from build123d import *
from build123d.topology import SkipClean

# Parameters (mm, degrees)
SKETCH1_R           = 15.24
SKETCH1_R_2         = 14.01445
BOSS_EXTRUDE1_DEPTH = 19.304
SKETCH2_R           = 14.01445
CUT_EXTRUDE1_DEPTH  = 29.934204707
CUT_EXTRUDE2_DEPTH  = 29.934204707
BOSS_EXTRUDE2_START = 1.27
BOSS_EXTRUDE2_DEPTH = 1.27
SKETCH6_R           = 4.699
CUT_EXTRUDE3_DEPTH  = 29.934204707
SKETCH8_W           = 17.272
SKETCH8_H           = 8.89
SKETCH8_R           = 2.54
BOSS_EXTRUDE3_DEPTH = 2.54
SKETCH9_W           = 2.159
SKETCH9_H           = 7.112
CUT_EXTRUDE4_DEPTH  = 1.27


with BuildPart() as part:
    # Sketch1 → Boss-Extrude1 (new body)
    # profile 1 of 2: a face of its own
    with BuildSketch(Plane(origin=(0, 0, 0), x_dir=(1, 0, 0), z_dir=(0, 1, 0))):
        Circle(SKETCH1_R)
        Circle(SKETCH1_R_2, mode=Mode.SUBTRACT)
    # profile 2 of 2: a face of its own
    with BuildSketch(Plane(origin=(0, 0, 0), x_dir=(1, 0, 0), z_dir=(0, 1, 0))):
        Polygon((-9.525, -12.563180017), (-10.16, -9.652937833), (10.16, -9.652937833), (9.525, -12.563180017), (9.525, -15.240937833), (-9.525, -15.240937833), align=None)
    extrude(amount=BOSS_EXTRUDE1_DEPTH)

    # Sketch2 → Cut-Extrude1 (cut, through all)
    with BuildSketch(Plane(origin=(0, 19.304, 0), x_dir=(1, 0, 0), z_dir=(0, 1, 0))):
        with Locations(Location((0, 0, 0), (0, 0, 270))):
            Circle(SKETCH2_R)
    extrude(amount=-CUT_EXTRUDE1_DEPTH, mode=Mode.SUBTRACT)

    # Sketch3 → Cut-Extrude2 (cut, through all)
    with SkipClean():  # the faces are left unmerged after this step: merging them gives an invalid solid
        with BuildSketch(Plane(origin=(0, 19.304, 0), x_dir=(1, 0, 0), z_dir=(0, 1, 0))):
            with BuildLine():
                Line((-8.636, -14.01445), (-8.636, -15.240937833))
                Line((-8.636, -15.240937833), (8.636, -15.240937833))
                Line((8.636, -15.240937833), (8.636, -14.01445))
                Line((8.636, -14.01445), (8.636, -11.037405166))
                ThreePointArc((8.636, -11.037405166), (0, -14.01445), (-8.636, -11.037405166))
                Line((-8.636, -11.037405166), (-8.636, -14.01445))
            make_face()
        extrude(amount=-CUT_EXTRUDE2_DEPTH, mode=Mode.SUBTRACT)

    # Sketch4 → Boss-Extrude2 (add)
    with SkipClean():  # the faces are left unmerged after this step: merging them gives an invalid solid
        with BuildSketch(Plane.XZ.offset(BOSS_EXTRUDE2_START)):
            with BuildLine():
                Line((9.525, 12.563180017), (9.701775888, 11.753005769))
                ThreePointArc((9.701775888, 11.753005769), (0, -15.24), (-9.701775888, 11.753005769))
                Line((-9.701775888, 11.753005769), (-9.525, 12.563180017))
                Line((-9.525, 12.563180017), (9.525, 12.563180017))
            make_face()
        extrude(amount=-BOSS_EXTRUDE2_DEPTH)

    # Sketch6 → Cut-Extrude3 (cut, through all)
    with BuildSketch(Plane.XZ):
        with Locations((0, -9.534819983)):
            Circle(SKETCH6_R)
    extrude(amount=-CUT_EXTRUDE3_DEPTH, mode=Mode.SUBTRACT)

    # Sketch8 → Boss-Extrude3 (add)
    # profile 1 of 2: a face of its own
    with BuildSketch(Plane.XZ.offset(1.27)):
        with Locations((23.114, 0)):
            Rectangle(SKETCH8_W, SKETCH8_H)
        with Locations(Location((23.114, 0, 0), (0, 0, 270))):
            Circle(SKETCH8_R, mode=Mode.SUBTRACT)
    # profile 2 of 2: a face of its own
    with BuildSketch(Plane.XZ.offset(1.27)):
        with Locations((-23.114, 0)):
            Rectangle(SKETCH8_W, SKETCH8_H)
        with Locations(Location((-23.114, 0, 0), (0, 0, 90))):
            Circle(SKETCH8_R, mode=Mode.SUBTRACT)
    extrude(amount=-BOSS_EXTRUDE3_DEPTH)

    # Sketch9 → Cut-Extrude4 (cut)
    with BuildSketch(Plane(origin=(0, 19.304, 0), x_dir=(1, 0, 0), z_dir=(0, 1, 0))):
        with Locations((14.605, 0)):
            Rectangle(SKETCH9_W, SKETCH9_H)
        with Locations((-14.605, 0)):
            Rectangle(SKETCH9_W, SKETCH9_H)
    extrude(amount=-CUT_EXTRUDE4_DEPTH, mode=Mode.SUBTRACT)


solid = part.part
Model file for the job. Use its own axes, mm. A direction names the side the tool comes from. Round coordinates to 2 decimals unless told otherwise and drop trailing zeros. Order: outer loops, then holes, each group sorted by start corner. A loop starts at its lowest first (then second) coordinate and runs counter-clockwise, first axis right, second up.
(1) Band-saw the part on A-A (z = -0.5). List the corners of the cut face in (x, y).
(2) Pin check, flat tips, straight feed: pin 1 (3 mm diameter, centred on x = 24, y = 0.5, fed in from -Z) (3 decimals); pin 2 (1.4 mm diameter, centred on x = 14.5, y = 18.5, fed in from +Z); pin 3 (12 mm diameter, centred on x = 1.5, y = 14.5, fed in from +Z); pin 4 (4.5 mm diameter, centred on x = -23, z = 0, fed in from +Y). Stop position of each tip, or through.
(3) Band-saw the part on B-B (y = 7.75). List the corners of the cut face in (x, z) (3 decimals), then the cut area to 3 significant figures.
(4) Band-saw the part on D-D (z = -6). List the corners of the cut face in (x, y), then the cut area to 3 significant figures.
(5) Pull direction Z, two halves, no side cores. Call faces 6 (the face through (31.75, 0, 0)), 7 (the face through (23, 0, -4.445)), 8 (the face through (14, 19, 3.556)), 9 (the face through (23, 0, 4.445)): released by +Z, released by -Z, zero draft, split by the parting line, or undercut.
(6) Band-saw the part on C-C (x = 0). List the corners of the cut face in (y, z), then the cut area to 3 significant figures.
(7) Drill centre lines: line 1 (X direction, y = -0.5, z = 0); line 2 (X direction, y = 0.5, z = 0); line 3 (X direction, y = 8.5, z = 12.5). Where is each one in solid material? Low to high.
(8) 3-axis set-ups, long thin cutter, end or side, ignore diameter. For faces 1 (the face through (0, 0, -1)), 2 (the face through (14, 19, -3.556)), 3 (the face through (9.525, 10, 14)), 4 (the face through (-23, 0, 4.445)), 5 (the face through (8.636, 10, 13)): which of +Z, -Z, +X, -X, +Y, -Y reach the whole face in a straight line?
Verdict:
1. outline: (-31.75, -1.27) - (-25.6, -1.27) - (-25.6, 1.27) - (-31.75, 1.27) - close; (-20.62, -1.27) - (20.62, -1.27) - (20.62, 1.27) - (15.23, 1.27) - (15.23, 18.03) - (14.01, 18.03) - (14.01, 0) - (-14.01, 0) - (-14.01, 18.03) - (-15.23, 18.03) - (-15.23, 1.27) - (-20.62, 1.27) - close; (25.6, -1.27) - (31.75, -1.27) - (31.75, 1.27) - (25.6, 1.27) - close
2. pin 1: stops at z = -4.445
2. pin 2: stops at z = 6.47
2. pin 3: stops at z = -11.84
2. pin 4: passes through
3. outline: (-9.702, 11.753) arc R15.24 ccw (long way) to (9.702, 11.753) - (9.525, 12.563) - (9.525, 15.241) - (8.636, 15.241) - (8.636, 11.037) arc R14.014 cw to (1.717, -13.909) arc R4.699 cw to (-1.717, -13.909) arc R14.014 cw to (-8.636, 11.037) - (-8.636, 15.241) - (-9.525, 15.241) - (-9.525, 12.563) - close
3. area: 94.9 mm2
4. outline: (-14.01, -1.27) - (14.01, -1.27) - (14.01, 19.3) - (12.67, 19.3) - (12.67, 0) - (-12.67, 0) - (-12.67, 19.3) - (-14.01, 19.3) - close
4. area: 87.5 mm2
5. face 6: zero draft
5. face 7: released by -Z
5. face 8: undercut
5. face 9: released by +Z
6. outline: (-1.27, -15.24) - (19.3, -15.24) - (19.3, -14.23) - (0, -14.23) - (0, 12.56) - (-1.27, 12.56) - close
6. area: 54.7 mm2
7. line 1: x = -31.75 to -25.65, -20.57 to 20.57, 25.65 to 31.75
7. line 2: x = -31.75 to -25.65, -20.57 to -14.01, 14.01 to 20.57, 25.65 to 31.75
7. line 3: x = -9.54 to -8.64, 8.64 to 9.54
8. face 1: +Y
8. face 2: +X, -X, +Y
8. face 3: +Z, +X, +Y, -Y
8. face 4: +Z, -X, +Y, -Y
8. face 5: +Z, +Y
